Work out the finished part from the listing and answer in its coordinate system (mm). A direction names the side the tool comes from. Give positions to 0.01 mm unless a question says otherwise; leave off trailing zeros. Order: outer loops, then holes, each group sorted by start corner. A loop starts at its lowest first (then second) coordinate and runs counter-clockwise, first axis right, second up. Notation, with made-up numbers: (11.5, -37) -> (43.5, -37) arc R27 ccw to (43.5, -6) -> close; hole circle Ø1 at (80.5, 82.5). An arc over 180 degrees is marked (long way). Answer as CSV lines item,"result". Start each with the question number.
1. Find the intervals of material crossed by L1, parallel to Z at x = -91.5, y = 65; L2, parallel to Y at x = -21, z = 6.25; L3, parallel to Y at x = 85, z = 12.5, in increasing order.
2. For faces 1 (the flat face through (1, 71.625, 4)), 2 (the flat face through (-159.225, 69, 12)), determine the directions among +Z, -Z, +X, -X, +Y, -Y from which every point of the face is accessible in a straight line to the end or side of a thin tool.
3. A cutting plane is placed at B-B (z = 4.75). Give the vertices of the cut face in (x, y), then the cut area to 3 significant figures.
4. A cutting plane is placed at A-A (x = 23.5). Give the vertices of the cut face in (y, z).
5. Flat-ended cylindrical pins translate along their axes: pin 1 (4.5 mm diameter, centred on y = 45.5, z = 11.5, fed in from -X); pin 2 (8 mm diameter, centred on x = 121, y = 55, fed in from -Z); pin 3 (3.5 mm diameter, centred on x = -65.78, y = 67.12, fed in from -Z); pin 4 (3 mm diameter, centred on x = -8, z = 12.5, fed in from -Y). Find the tip coordinate at first contact, or state that the pin passes through.
6. A cutting plane is placed at D-D (x = 140.5). Give the vertices of the cut face in (y, z).
7. A cutting plane is placed at C-C (y = 52.5). Give the vertices of the cut face in (x, z).
from build123d import *

# Parameters (mm, degrees)
BOSS_EXTRUDE1_DEPTH                          = 4
SKETCH3_W                                    = 324.79935
SKETCH3_H                                    = 12
BOSS_EXTRUDE2_DEPTH                          = 2
FILLET1_SIZE                                 = 1
FILLET2_R                                    = 1.6
FILLET3_R                                    = 12
TAP_DRILL_FOR_M3X0_5_TAP1_D                  = 2.5
TAP_DRILL_FOR_M3X0_5_TAP1_DEPTH              = 7
TAP_DRILL_FOR_M3X0_5_TAP1_CSINK_D            = 2.55
TAP_DRILL_FOR_M3X0_5_TAP1_CSINK_ANGLE        = 90
TAP_DRILL_FOR_M3X0_5_TAP1_TIP                = 0.751075774
CBORE_FOR_M2_5_HEX_SOCKET_HEAD_CAP_S_2_COUNT = 2
CBORE_FOR_M2_5_HEX_SOCKET_HEAD_CAP_S_2_PITCH = 343.798403
CBORE_FOR_M2_5_HEX_SOCKET_HEAD_CAP_S_3_COUNT = 2
CBORE_FOR_M2_5_HEX_SOCKET_HEAD_CAP_S_3_PITCH = 369.079907741
CBORE_FOR_M2_5_HEX_SOCKET_HEAD_CAP_S_4_COUNT = 2
CBORE_FOR_M2_5_HEX_SOCKET_HEAD_CAP_S_4_PITCH = 275.745768266
CBORE_FOR_M2_5_HEX_SOCKET_HEAD_CAP_S_5_COUNT = 2
CBORE_FOR_M2_5_HEX_SOCKET_HEAD_CAP_S_5_PITCH = 169.171931368
CBORE_FOR_M2_5_HEX_SOCKET_HEAD_CAP_S_6_COUNT = 2
CBORE_FOR_M2_5_HEX_SOCKET_HEAD_CAP_S_6_PITCH = 134.248413


with BuildPart() as part:
    # Sketch2 → Boss-Extrude1 (new body)
    with BuildSketch(Plane.XY.offset(14.1038)):
        Polygon((-159.224575, 59.6246), (-159.224575, 73.6246), (165.574775, 73.6246), (165.574775, 59.6246), (165.574775, 40.6744), (148.575775, 40.6744), (148.575775, 59.6246), align=None)
    extrude(amount=-BOSS_EXTRUDE1_DEPTH)

    # Sketch3 → Boss-Extrude2 (add)
    with BuildSketch(Plane(origin=(0, 73.6246, 0), x_dir=(1, 0, 0), z_dir=(0, 1, 0))):
        with Locations((3.1751, -4.1038)):
            Rectangle(SKETCH3_W, SKETCH3_H)
    extrude(amount=-BOSS_EXTRUDE2_DEPTH)

    # Fillet1
    fillet1_edges = [part.edges().sort_by_distance(p)[0] for p in [
        (3.1751, 73.6246, 14.1038),
    ]]
    chamfer(fillet1_edges, length=FILLET1_SIZE)

    # Fillet2
    fillet2_edges = [part.edges().sort_by_distance(p)[0] for p in [
        (165.574775, 40.6744, 12.1038),
        (148.575775, 40.6744, 12.1038),
        (-159.224575, 59.6246, 12.1038),
        (165.574775, 72.6246, -1.8962),
        (-159.224575, 72.6246, -1.8962),
    ]]
    fillet(fillet2_edges, radius=FILLET2_R)

    # Fillet3
    fillet3_edges = [part.edges().sort_by_distance(p)[0] for p in [
        (148.575775, 59.6246, 12.1038),
    ]]
    fillet(fillet3_edges, radius=FILLET3_R)

    # Tap Drill for M3x0.5 Tap1
    with Locations(Plane(origin=(0, 0, 5.0798), x_dir=(-1, 0, 0), z_dir=(0, 0, -1))):
        with Locations((-106.614905, 66.623653), (-37.655035, 66.623653), (31.304835, 66.623653), (100.264705, 66.623653), (100.264705, -66.62476), (31.304835, -66.62476), (-37.655035, -66.62476), (-106.614905, -66.62476)):
            CounterSinkHole(TAP_DRILL_FOR_M3X0_5_TAP1_D / 2, TAP_DRILL_FOR_M3X0_5_TAP1_CSINK_D / 2, depth=TAP_DRILL_FOR_M3X0_5_TAP1_DEPTH, counter_sink_angle=TAP_DRILL_FOR_M3X0_5_TAP1_CSINK_ANGLE)
            with Locations((0, 0, -(TAP_DRILL_FOR_M3X0_5_TAP1_DEPTH + TAP_DRILL_FOR_M3X0_5_TAP1_TIP / 2))):  # 118° drill point
                Cone(0, TAP_DRILL_FOR_M3X0_5_TAP1_D / 2, TAP_DRILL_FOR_M3X0_5_TAP1_TIP, mode=Mode.SUBTRACT)

    # Sketch7 → CBORE for M2.5 Hex Socket Head Cap Screw1 (revolve, cut)
    with BuildSketch(Plane(origin=(-168.7241015, -67.1242865, -6), x_dir=(0, 1, 0), z_dir=(1, 0, 0))):
        Polygon((0, 0), (0, 18.871247898), (1.45, 18), (1.45, 5.9), (2.75, 5.9), (2.75, 0.025), (2.775, 0), align=None)
    cbore_for_m2_5_hex_socket_head_cap_screw = revolve(axis=Axis((-168.7241015, -67.1242865, -12.35), (0, 0, 1)), mode=Mode.SUBTRACT)

    # CBORE for M2.5 Hex Socket Head Cap S 2: CBORE for M2.5 Hex Socket Head Cap Screw1 ×2
    with Locations(*[(i * CBORE_FOR_M2_5_HEX_SOCKET_HEAD_CAP_S_2_PITCH, 0, 0) for i in range(1, CBORE_FOR_M2_5_HEX_SOCKET_HEAD_CAP_S_2_COUNT)]):
        add(cbore_for_m2_5_hex_socket_head_cap_screw, mode=Mode.SUBTRACT)

    # CBORE for M2.5 Hex Socket Head Cap S 3: CBORE for M2.5 Hex Socket Head Cap Screw1 ×2
    with Locations(*[Vector(0.9315012705620509, 0.3637380691394355, 0) * (i * CBORE_FOR_M2_5_HEX_SOCKET_HEAD_CAP_S_3_PITCH) for i in range(1, CBORE_FOR_M2_5_HEX_SOCKET_HEAD_CAP_S_3_COUNT)]):
        add(cbore_for_m2_5_hex_socket_head_cap_screw, mode=Mode.SUBTRACT)

    # CBORE for M2.5 Hex Socket Head Cap S 4: CBORE for M2.5 Hex Socket Head Cap Screw1 ×2
    with Locations(*[Vector(0.873482385656236, 0.48685575065751296, 0) * (i * CBORE_FOR_M2_5_HEX_SOCKET_HEAD_CAP_S_4_PITCH) for i in range(1, CBORE_FOR_M2_5_HEX_SOCKET_HEAD_CAP_S_4_COUNT)]):
        add(cbore_for_m2_5_hex_socket_head_cap_screw, mode=Mode.SUBTRACT)

    # CBORE for M2.5 Hex Socket Head Cap S 5: CBORE for M2.5 Hex Socket Head Cap Screw1 ×2
    with Locations(*[Vector(0.6084894265127476, 0.7935619810841417, 0) * (i * CBORE_FOR_M2_5_HEX_SOCKET_HEAD_CAP_S_5_PITCH) for i in range(1, CBORE_FOR_M2_5_HEX_SOCKET_HEAD_CAP_S_5_COUNT)]):
        add(cbore_for_m2_5_hex_socket_head_cap_screw, mode=Mode.SUBTRACT)

    # CBORE for M2.5 Hex Socket Head Cap S 6: CBORE for M2.5 Hex Socket Head Cap Screw1 ×2
    with Locations(*[(0, i * CBORE_FOR_M2_5_HEX_SOCKET_HEAD_CAP_S_6_PITCH, 0) for i in range(1, CBORE_FOR_M2_5_HEX_SOCKET_HEAD_CAP_S_6_COUNT)]):
        add(cbore_for_m2_5_hex_socket_head_cap_screw, mode=Mode.SUBTRACT)


solid = part.part
Answer sheet:
1,L1,"z = 10.1 to 14.1"
1,L2,"y = 71.62 to 73.62"
1,L3,"y = 59.62 to 73.62"
2,face 1,"-Z, +X, -X, -Y"
2,face 2,"+Z, -Z, -X, +Y, -Y"
3,outline,"(-159.22, 71.62) -> (165.57, 71.62) -> (165.57, 73.62) -> (-159.22, 73.62) -> close"
3,area,"650 mm^2"
4,outline,"(59.62, 10.1) -> (71.62, 10.1) -> (71.62, -1.9) -> (73.62, -1.9) -> (73.62, 13.1) -> (72.62, 14.1) -> (59.62, 14.1) -> close"
5,pin 1,"stops at x = 148.58"
5,pin 2,"passes through"
5,pin 3,"stops at z = 10.1"
5,pin 4,"stops at y = 59.62"
6,outline,"(58.96, 10.1) -> (71.62, 10.1) -> (71.62, -1.9) -> (73.62, -1.9) -> (73.62, 13.1) -> (72.62, 14.1) -> (58.96, 14.1) -> close"
7,outline,"(147.54, 10.1) -> (165.57, 10.1) -> (165.57, 14.1) -> (147.54, 14.1) -> close"
